from build123d import *

# Parameters (mm, degrees)
MAGNET_OUTER_DIM_R  = 5
BOSS_EXTRUDE7_DEPTH = 2.5
CUT_EXTRUDE1_START  = 0.3
MAGNET_DIM_R        = 3
CUT_EXTRUDE1_DEPTH  = 2.2
MOTOTR_OUTER_DIM_R  = 7
BOSS_EXTRUDE8_DEPTH = 2.5
CUT_EXTRUDE4_START  = -3.4
MOTOR_DIM_R         = 5
CUT_EXTRUDE4_DEPTH  = 3.2


with BuildPart() as part:
    # magnet_outer_dim → Boss-Extrude7 (new body)
    with BuildSketch(Plane(origin=(0, 0, 0), x_dir=(1, 0, 0), z_dir=(0, 1, 0))):
        with Locations(Location((0, 0, 0), (0, 0, 270))):
            Circle(MAGNET_OUTER_DIM_R)
    extrude(amount=BOSS_EXTRUDE7_DEPTH)

    # magnet_dim → Cut-Extrude1 (cut)
    with BuildSketch(Plane(origin=(0, 0, 0), x_dir=(1, 0, 0), z_dir=(0, 1, 0)).offset(CUT_EXTRUDE1_START)):
        with Locations(Location((0, 0, 0), (0, 0, 270))):
            Circle(MAGNET_DIM_R)
    extrude(amount=CUT_EXTRUDE1_DEPTH, mode=Mode.SUBTRACT)

    # mototr_outer_dim → Boss-Extrude8 (add)
    with BuildSketch(Plane(origin=(0, 0, 0), x_dir=(1, 0, 0), z_dir=(0, 1, 0))):
        with Locations(Location((0, 0, 0), (0, 0, 270))):
            Circle(MOTOTR_OUTER_DIM_R)
    extrude(amount=-BOSS_EXTRUDE8_DEPTH)

    # motor_dim → Cut-Extrude4 (cut)
    with BuildSketch(Plane(origin=(0, 0, 0), x_dir=(1, 0, 0), z_dir=(0, 1, 0)).offset(CUT_EXTRUDE4_START)):
        with Locations(Location((0, 0, 0), (0, 0, 270))):
            Circle(MOTOR_DIM_R)
    extrude(amount=CUT_EXTRUDE4_DEPTH, mode=Mode.SUBTRACT)


solid = part.part
Work out the finished part from the listing and answer in its coordinate system (mm). A direction names the side the tool comes from. Give positions to 0.01 mm unless a question says otherwise; leave off trailing zeros. Order: outer loops, then holes, each group sorted by start corner. A loop starts at its lowest first (then second) coordinate and runs counter-clockwise, first axis right, second up. Notation, with made-up numbers: (48.5, 6) -> (89.5, 6) arc R19 ccw to (89.5, 33) -> close; hole circle Ø10 at (3.25, 89.25). An arc over 180 degrees is marked (long way). Answer as a JSON object with one key per item and string values. Group by question number.
1. Consider line 1 along Y through (x, z) = (-4.5, 0.5); line 2 along Y through (x, z) = (2.75, -5.75); line 3 along X through (y, z) = (-1.25, -1.25). Determine where each line is inside the solid, lowest interval first. Write a range as [from, to].
2. Flat-ended cylindrical pins translate along their axes: pin 1 Ø1.5 at (y, z) = (-1, 5.5) entering from -X; pin 2 Ø1 at (x, z) = (0, 3) entering from -Y. Find the tip coordinate at first contact, or state that the pin passes through.
3. Section B-B on y = 2.1 is taken. Determine the outline of the cut face in (x, z), plus the area to 3 significant figures.
4. Section A-A on x = 0 is taken. Determine the outline of the cut face in (y, z).
5. The mould has two halves that part along Z. Classify faces 4 (the cylindrical face through (-4.88, -1.37, -1.08)), 5 (the flat face through (-3.3, 2.5, -0.1)), 6 (the cylindrical face through (-4.88, 1.23, -1.08)): released by +Z, released by -Z, zero draft, split by the parting line, or undercut.
6. Section C-C on z = -2.25 is taken. Determine the outline of the cut face in (x, y).
7. Section D-D on y = -1.7 is taken. Determine the outline of the cut face in (x, z).
8. A tool of negligible diameter and unlimited length cuts with its end or side. For faces 1 (the flat face through (0, -0.2, 0)), 2 (the flat face through (5, -2.5, -2)), 3 (the flat face through (0, 0.3, 0)), from which of +Z, -Z, +X, -X, +Y, -Y can it reach the whole face along a straight path? Write none if from no direction.
Result sheet:
{
 "1": {"line 1": "y = [-0.2, 2.5]", "line 2": "y = [-2.5, 0]", "line 3": "x = [-6.89, -4.84], [4.84, 6.89]"},
 "2": {"pin 1": "stops at x = -5.14", "pin 2": "stops at y = -0.2"},
 "3": {"outline": "circle Ø10 at (0, 0); hole circle Ø6 at (0, 0)", "area": "50.3 mm^2"},
 "4": {"outline": "(-2.5, -7) -> (0, -7) -> (0, -5) -> (2.5, -5) -> (2.5, -3) -> (0.3, -3) -> (0.3, 3) -> (2.5, 3) -> (2.5, 5) -> (0, 5) -> (0, 7) -> (-2.5, 7) -> (-2.5, 5) -> (-0.2, 5) -> (-0.2, -5) -> (-2.5, -5) -> close"},
 "5": {"face 4": "undercut", "face 5": "zero draft", "face 6": "split by the parting line"},
 "6": {"outline": "(-6.63, -2.5) -> (-4.47, -2.5) -> (-4.47, -0.2) -> (4.47, -0.2) -> (4.47, -2.5) -> (6.63, -2.5) -> (6.63, 0) -> (4.47, 0) -> (4.47, 2.5) -> (1.98, 2.5) -> (1.98, 0.3) -> (-1.98, 0.3) -> (-1.98, 2.5) -> (-4.47, 2.5) -> (-4.47, 0) -> (-6.63, 0) -> close"},
 "7": {"outline": "circle Ø14 at (0, 0); hole circle Ø10 at (0, 0)"},
 "8": {"face 1": "-Y", "face 2": "+Z, -Z, +X, -X, -Y", "face 3": "+Y"}
}
